Geometry: final body of the model. Coordinates: model frame, mm. A direction names the side the tool comes from. Coordinates: 2 decimals unless noted, no trailing zeros. Loops run counter-clockwise (first coordinate to the right, second up) from the corner with the lowest first, then second, coordinate; pieces in that order, holes last. Notation, with made-up numbers: (-13.75, 6.5) - (-9.75, 6.5) arc R25 cw to (-9.75, 22.5) - close; hole circle Ø9 at (6.25, -8). An arc over 180 degrees is marked (long way). Write each question's results on one line, items separated by ' | '. Start each with the question number.
from build123d import *

# Parameters (mm, degrees)
SKETCH1_W            = 281.94
SKETCH1_H            = 228.6
BOSS_EXTRUDE2_DEPTH  = 25.4
SKETCH3_W            = 281.94
SKETCH3_H            = 17.526
CUT_EXTRUDE1_DEPTH   = 8.128
SKETCH4_W            = 11.43
SKETCH4_H            = 211.074
BOSS_EXTRUDE4_DEPTH  = 3.175
SKETCH5_W            = 278.765
SKETCH5_H            = 11.43
BOSS_EXTRUDE9_DEPTH  = 3.175
SKETCH9_W            = 11.43
SKETCH9_H            = 207.899
BOSS_EXTRUDE10_DEPTH = 3.175
SKETCH8_W            = 281.94
SKETCH8_H            = 11.43
BOSS_EXTRUDE11_DEPTH = 3.175
SKETCH10_W           = 281.94
SKETCH10_H           = 14.351
CUT_EXTRUDE2_DEPTH   = 10.16
SKETCH11_W           = 275.59
SKETCH11_H           = 207.899
CUT_EXTRUDE3_DEPTH   = 10.16
CUT_EXTRUDE4_DEPTH   = 10.16
SKETCH13_W           = 281.94
SKETCH13_H           = 3.175
CUT_EXTRUDE5_DEPTH   = 10.16
SHELL4_START         = -65.823170732
SHELL4_DEPTH         = 276.86


# Read off the part's stored shape, not the designer's step: Shell4
with BuildPart() as part:
    # Sketch1 → Boss-Extrude2 (new body)
    with BuildSketch(Plane.XY):
        with Locations((72.606829268, 16.339634146)):
            Rectangle(SKETCH1_W, SKETCH1_H)
    extrude(amount=BOSS_EXTRUDE2_DEPTH)

    # Sketch3 → Cut-Extrude1 (cut)
    with BuildSketch(Plane.XY.offset(25.4)):
        with Locations((72.606829268, -89.197365854)):
            Rectangle(SKETCH3_W, SKETCH3_H)
    extrude(amount=-CUT_EXTRUDE1_DEPTH, mode=Mode.SUBTRACT)



with BuildPart() as body_2:
    # Sketch4 → Boss-Extrude4 (new body)
    with BuildSketch(Plane.ZY.offset(68.363170732)):
        with Locations((31.115, 25.102634146)):
            Rectangle(SKETCH4_W, SKETCH4_H)
    extrude(amount=-BOSS_EXTRUDE4_DEPTH)


with BuildPart() as part_1:
    add(part.part)

    add(body_2.part)  # Boss-Extrude9 merges body 2
    # Sketch5 → Boss-Extrude9 (add)
    with BuildSketch(Plane(origin=(0, 130.639634146, 0), x_dir=(1, 0, 0), z_dir=(0, 1, 0))):
        with Locations((74.194329268, -31.115)):
            Rectangle(SKETCH5_W, SKETCH5_H)
    extrude(amount=-BOSS_EXTRUDE9_DEPTH)

    # Sketch9 → Boss-Extrude10 (add)
    with BuildSketch(Plane(origin=(213.576829268, 0, 0), x_dir=(0, 0, -1), z_dir=(1, 0, 0))):
        with Locations((-31.115, 23.515134146)):
            Rectangle(SKETCH9_W, SKETCH9_H)
    extrude(amount=-BOSS_EXTRUDE10_DEPTH)


with BuildPart() as body_2_2:
    # Sketch8 → Boss-Extrude11 (new body)
    with BuildSketch(Plane.XZ.offset(97.960365854)):
        with Locations((72.606829268, 22.987)):
            Rectangle(SKETCH8_W, SKETCH8_H)
    extrude(amount=-BOSS_EXTRUDE11_DEPTH)

    # Combine1: union part
    add(part_1.part)

    # Sketch10 → Cut-Extrude2 (cut)
    with BuildSketch(Plane.XY.offset(17.272)):
        with Locations((72.606829268, -87.609865854)):
            Rectangle(SKETCH10_W, SKETCH10_H)
    extrude(amount=-CUT_EXTRUDE2_DEPTH, mode=Mode.SUBTRACT)

    # Sketch11 → Cut-Extrude3 (cut)
    with BuildSketch(Plane.XY.offset(25.4)):
        with Locations((72.606829268, 23.515134146)):
            Rectangle(SKETCH11_W, SKETCH11_H)
    extrude(amount=-CUT_EXTRUDE3_DEPTH, mode=Mode.SUBTRACT)

    # Sketch12 → Cut-Extrude4 (cut)
    with BuildSketch(Plane.XY.offset(36.83)):
        Polygon((-68.363170732, -80.434365854), (-65.188170732, -80.434365854), (-65.188170732, 127.464634146), (210.401829268, 127.464634146), (210.401829268, -80.434365854), (213.576829268, -80.434365854), (213.576829268, 130.639634146), (-68.363170732, 130.639634146), align=None)
    extrude(amount=-CUT_EXTRUDE4_DEPTH, mode=Mode.SUBTRACT)

    # Sketch13 → Cut-Extrude5 (cut)
    with BuildSketch(Plane.XY.offset(28.702)):
        with Locations((72.606829268, -96.372865854)):
            Rectangle(SKETCH13_W, SKETCH13_H)
    extrude(amount=-CUT_EXTRUDE5_DEPTH, mode=Mode.SUBTRACT)

    # Shell4 outline → Shell4 (cut)
    with BuildSketch(Plane.YZ.offset(SHELL4_START)):
        Polygon((-95.420365854, 4.572), (-95.420365854, 2.54), (128.099634146, 2.54), (128.099634146, 12.7), (-77.894365854, 12.7), (-77.894365854, 4.572), align=None)
    extrude(amount=SHELL4_DEPTH, mode=Mode.SUBTRACT)


solid = body_2_2.part
1) Section query B-B on z = 21.75. Output: boundary loops of the cut face in (x, y), and give its area (3 significant figures).
2) Access query for faces 1 (the flat face through (71, -88, 7.112)), 2 (the flat face through (71, 25, 15.24)), 3 (the flat face through (71, 128.1, 8)). Directions: +Z, -Z, +X, -X, +Y, -Y. A direction counts if a zero-diameter tool reaches every point of the face in a straight line with its end or side. Return the directions, or none.
3) Section query A-A on y = -57.5. Output: boundary loops of the cut face in (x, z), and give its area (3 significant figures).
4) Section query C-C on x = 48.5. Output: boundary loops of the cut face in (y, z), and give its area (3 significant figures).
5) Pull-direction query (Y, two-part tool) for faces 4 (the flat face through (-65.188, 25, 21)), 5 (the flat face through (-68.363, 18, 13)), 6 (the flat face through (71, 130.64, 13)); classes: released by +Y, released by -Y, zero draft, split by the parting line, or undercut.
6) Pin query (flat end, axial travel): pin 1 Ø12 at (x, y) = (0, 43) entering from +Z; pin 2 Ø14 at (x, y) = (108.5, -91) entering from -Z; pin 3 Ø3 at (x, z) = (116.5, 21) entering from -Y; pin 4 Ø7 at (x, y) = (24, -86) entering from +Z. Return the tip coordinate at first contact, or that it passes through.
7) Material intervals for line 1 (Y direction, x = 196, z = 12.5); line 2 (Z direction, x = 202, y = -10.5); line 3 (X direction, y = -59, z = 15.5), sorted ascending. Write a range as [from, to].
Returned:
1) outline: (-68.36, -80.43) - (-65.19, -80.43) - (-65.19, 127.46) - (210.4, 127.46) - (210.4, -80.43) - (213.58, -80.43) - (213.58, 130.64) - (-68.36, 130.64) - close | area: 2,220 mm²
2) face 1: +Z, +X, -X | face 2: +Z | face 3: none
3) outline: (-68.36, 0) - (213.58, 0) - (213.58, 26.67) - (210.4, 26.67) - (210.4, 15.24) - (-65.19, 15.24) - (-65.19, 26.67) - (-68.36, 26.67) - close; hole (-65.82, 2.54) - (211.04, 2.54) - (211.04, 12.7) - (-65.82, 12.7) - close | area: 1,560 mm²
4) outline: (-97.96, 0) - (130.64, 0) - (130.64, 26.67) - (127.46, 26.67) - (127.46, 15.24) - (-80.43, 15.24) - (-80.43, 7.11) - (-94.79, 7.11) - (-94.79, 18.54) - (-97.96, 18.54) - close; hole (-95.42, 2.54) - (128.1, 2.54) - (128.1, 12.7) - (-77.89, 12.7) - (-77.89, 4.57) - (-95.42, 4.57) - close | area: 1,290 mm²
5) face 4: undercut | face 5: zero draft | face 6: released by +Y
6) pin 1: stops at z = 15.24 | pin 2: stops at z = 0 | pin 3: stops at y = 127.46 | pin 4: stops at z = 7.11
7) line 1: y = [-97.96, -94.79], [-80.43, -77.89], [128.1, 130.64] | line 2: z = [0, 2.54], [12.7, 15.24] | line 3: x = [-68.36, -65.19], [210.4, 213.58]
